from build123d import *

# Parameters (mm, degrees)
SKETCH1_R           = 1.5
SKETCH1_R_2         = 3
SKETCH1_R_3         = 12
SKETCH1_W           = 2.8
SKETCH1_H           = 30
BOSS_EXTRUDE4_DEPTH = 3


with BuildPart() as part:
    # Sketch1 → Boss-Extrude4 (new body)
    with BuildSketch(Plane(origin=(0, 0, 0), x_dir=(1, 0, 0), z_dir=(0, 1, 0))):
        with BuildLine():
            Line((-121.196449229, -126.808304592), (-11.829794241, -126.808304592))
            ThreePointArc((-11.829794241, -126.808304592), (9.383409194, -118.021508028), (18.170205759, -96.808304592))
            Line((18.170205759, -96.808304592), (18.170205759, -42.124977099))
            ThreePointArc((18.170205759, -42.124977099), (-66.513121735, 42.558350395), (-151.196449229, -42.124977099))
            Line((-151.196449229, -42.124977099), (-151.196449229, -96.808304592))
            ThreePointArc((-151.196449229, -96.808304592), (-142.409652664, -118.021508028), (-121.196449229, -126.808304592))
        make_face()
        with Locations(Location((-19.417066349, 12.133998526, 0), (0, 0, 270))):
            Circle(SKETCH1_R, mode=Mode.SUBTRACT)
        with Locations(Location((-19.417066349, -63.912266725, 0), (0, 0, 270))):
            Circle(SKETCH1_R, mode=Mode.SUBTRACT)
        with Locations(Location((-113.609177122, -63.912266725, 0), (0, 0, 270))):
            Circle(SKETCH1_R, mode=Mode.SUBTRACT)
        with Locations(Location((-113.609177122, 12.133998526, 0), (0, 0, 270))):
            Circle(SKETCH1_R, mode=Mode.SUBTRACT)
        with Locations(Location((-20.763121735, -6.941649605, 0), (0, 0, 270))):
            Circle(SKETCH1_R, mode=Mode.SUBTRACT)
        with Locations(Location((-112.263121735, -6.941649605, 0), (0, 0, 270))):
            Circle(SKETCH1_R, mode=Mode.SUBTRACT)
        with Locations(Location((-112.263121735, -51.941649605, 0), (0, 0, 270))):
            Circle(SKETCH1_R, mode=Mode.SUBTRACT)
        with Locations(Location((-66.513121735, -115.308304592, 0), (0, 0, 270))):
            Circle(SKETCH1_R_2, mode=Mode.SUBTRACT)
        with Locations(Location((8.170205759, -42.124977099, 0), (0, 0, 270))):
            Circle(SKETCH1_R, mode=Mode.SUBTRACT)
        with Locations(Location((-141.196449229, -42.124977099, 0), (0, 0, 270))):
            Circle(SKETCH1_R, mode=Mode.SUBTRACT)
        with Locations(Location((-66.513121735, 5.435278237, 0), (0, 0, 270))):
            Circle(SKETCH1_R_3, mode=Mode.SUBTRACT)
        with Locations(Location((-66.513121735, 25.558350395, 0), (0, 0, 270))):
            Circle(SKETCH1_R_2, mode=Mode.SUBTRACT)
        with Locations(Location((-66.513121735, -69.564721763, 0), (0, 0, 270))):
            Circle(SKETCH1_R_3, mode=Mode.SUBTRACT)
        with Locations(Location((-107.213121735, -116.69721419, 0), (0, 0, 270))):
            Circle(SKETCH1_R, mode=Mode.SUBTRACT)
        with Locations(Location((-25.813121735, -116.69721419, 0), (0, 0, 270))):
            Circle(SKETCH1_R, mode=Mode.SUBTRACT)
        with Locations(Location((-25.813121735, -57.29721419, 0), (0, 0, 270))):
            Circle(SKETCH1_R, mode=Mode.SUBTRACT)
        with Locations(Location((-123.013121735, -10.138406212, 0), (0, 0, 270))):
            Circle(SKETCH1_R, mode=Mode.SUBTRACT)
        with Locations(Location((-107.213121735, -57.29721419, 0), (0, 0, 270))):
            Circle(SKETCH1_R, mode=Mode.SUBTRACT)
        with Locations(Location((-114.013120412, -46.008407352, 0), (0, 0, 270))):
            Circle(SKETCH1_R, mode=Mode.SUBTRACT)
        with Locations(Location((-19.013119912, -46.008407352, 0), (0, 0, 270))):
            Circle(SKETCH1_R, mode=Mode.SUBTRACT)
        with Locations(Location((-19.013119912, -103.708406252, 0), (0, 0, 270))):
            Circle(SKETCH1_R, mode=Mode.SUBTRACT)
        with Locations(Location((-114.013120412, -103.708406252, 0), (0, 0, 270))):
            Circle(SKETCH1_R, mode=Mode.SUBTRACT)
        with Locations(Location((-10.013121735, -10.138406212, 0), (0, 0, 270))):
            Circle(SKETCH1_R, mode=Mode.SUBTRACT)
        with Locations(Location((-10.013121735, -121.478406212, 0), (0, 0, 270))):
            Circle(SKETCH1_R, mode=Mode.SUBTRACT)
        with Locations(Location((-123.013121735, -121.478406212, 0), (0, 0, 270))):
            Circle(SKETCH1_R, mode=Mode.SUBTRACT)
        with Locations(Location((-125.513121735, -116.69721419, 0), (0, 0, 270))):
            Circle(SKETCH1_R, mode=Mode.SUBTRACT)
        with Locations(Location((-125.513121735, -45.59721419, 0), (0, 0, 270))):
            Circle(SKETCH1_R, mode=Mode.SUBTRACT)
        with Locations(Location((-7.513121735, -116.69721419, 0), (0, 0, 270))):
            Circle(SKETCH1_R, mode=Mode.SUBTRACT)
        with Locations(Location((-7.513121735, -45.59721419, 0), (0, 0, 270))):
            Circle(SKETCH1_R, mode=Mode.SUBTRACT)
        with Locations(Location((-80.013121735, 38.378834062, 0), (0, 0, 270))):
            Circle(SKETCH1_R, mode=Mode.SUBTRACT)
        with Locations(Location((-80.013121735, -19.621165938, 0), (0, 0, 270))):
            Circle(SKETCH1_R, mode=Mode.SUBTRACT)
        with Locations(Location((-31.013121735, -19.621165938, 0), (0, 0, 270))):
            Circle(SKETCH1_R, mode=Mode.SUBTRACT)
        with Locations(Location((-27.513121735, -72.508406212, 0), (0, 0, 270))):
            Circle(SKETCH1_R, mode=Mode.SUBTRACT)
        with Locations(Location((-27.513121735, -121.508406212, 0), (0, 0, 270))):
            Circle(SKETCH1_R, mode=Mode.SUBTRACT)
        with Locations(Location((-85.513121735, -72.508406212, 0), (0, 0, 270))):
            Circle(SKETCH1_R, mode=Mode.SUBTRACT)
        with Locations(Location((-85.513121735, -121.508406212, 0), (0, 0, 270))):
            Circle(SKETCH1_R, mode=Mode.SUBTRACT)
        with Locations(Location((-42.013121735, -100.008406212, 0), (0, 0, 270))):
            Circle(SKETCH1_R, mode=Mode.SUBTRACT)
        with Locations(Location((-91.013121735, -100.008406212, 0), (0, 0, 270))):
            Circle(SKETCH1_R, mode=Mode.SUBTRACT)
        with Locations(Location((-42.013121735, -42.008406212, 0), (0, 0, 270))):
            Circle(SKETCH1_R, mode=Mode.SUBTRACT)
        with Locations(Location((-91.013121735, -42.008406212, 0), (0, 0, 270))):
            Circle(SKETCH1_R, mode=Mode.SUBTRACT)
        with Locations(Location((-66.513121735, -109.124977099, 0), (0, 0, 270))):
            Circle(SKETCH1_R, mode=Mode.SUBTRACT)
        with Locations(Location((-66.513121735, -24.124977099, 0), (0, 0, 270))):
            Circle(SKETCH1_R, mode=Mode.SUBTRACT)
        with Locations(Location((-24.013121735, -66.624977099, 0), (0, 0, 270))):
            Circle(SKETCH1_R, mode=Mode.SUBTRACT)
        with Locations(Location((-109.013121735, -66.624977099, 0), (0, 0, 270))):
            Circle(SKETCH1_R, mode=Mode.SUBTRACT)
        with Locations(Location((-141.196449229, -109.124977099, 0), (0, 0, 270))):
            Circle(SKETCH1_R, mode=Mode.SUBTRACT)
        with Locations(Location((8.170205759, -109.124977099, 0), (0, 0, 270))):
            Circle(SKETCH1_R, mode=Mode.SUBTRACT)
        with Locations(Location((-20.763121735, -51.941649605, 0), (0, 0, 270))):
            Circle(SKETCH1_R, mode=Mode.SUBTRACT)
        with BuildLine():
            Line((-139.496449229, -88.862296701), (-139.496449229, -62.387657497))
            ThreePointArc((-139.496449229, -62.387657497), (-141.196449229, -60.687657497), (-142.896449229, -62.387657497))
            Line((-142.896449229, -62.387657497), (-142.896449229, -88.862296701))
            ThreePointArc((-142.896449229, -88.862296701), (-141.196449229, -90.562296701), (-139.496449229, -88.862296701))
        make_face(mode=Mode.SUBTRACT)
        with BuildLine():
            Line((-78.513121735, -120.108304592), (-54.513121735, -120.108304592))
            ThreePointArc((-54.513121735, -120.108304592), (-52.813121735, -121.808304592), (-54.513121735, -123.508304592))
            Line((-54.513121735, -123.508304592), (-78.513121735, -123.508304592))
            ThreePointArc((-78.513121735, -123.508304592), (-80.213121735, -121.808304592), (-78.513121735, -120.108304592))
        make_face(mode=Mode.SUBTRACT)
        with Locations((-14.413121735, -25.911649605)):
            Rectangle(SKETCH1_W, SKETCH1_H, mode=Mode.SUBTRACT)
        with Locations((-118.613121735, -25.911649605)):
            Rectangle(SKETCH1_W, SKETCH1_H, mode=Mode.SUBTRACT)
        with BuildLine():
            Line((9.870205759, -88.862296701), (9.870205759, -62.387657497))
            ThreePointArc((9.870205759, -62.387657497), (8.170205759, -60.687657497), (6.470205759, -62.387657497))
            Line((6.470205759, -62.387657497), (6.470205759, -88.862296701))
            ThreePointArc((6.470205759, -88.862296701), (8.170205759, -90.562296701), (9.870205759, -88.862296701))
        make_face(mode=Mode.SUBTRACT)
    extrude(amount=BOSS_EXTRUDE4_DEPTH)


solid = part.part
Can you work these out from the model? Positions are in its coordinate system, mm. Round coordinates to 2 decimals unless told otherwise and drop trailing zeros. Order: outer loops, then holes, each group sorted by start corner. A loop starts at its lowest first (then second) coordinate and runs counter-clockwise, first axis right, second up. Notation, with made-up numbers: M 73.25,83 L 98.25,83 A16 ccw 98.25,108 Z; hole C 29,-4 d2. An arc over 180 degrees is marked long. Use a Markdown table: item, result.
1) If we mould it in two halves opening along Z, with no side actions, what happens to faces 1 (the face through (9.1, 1.5, 118.3)), 2 (the face through (-78.228, 1.479, -8.037)), 3 (the face through (-68, 3, 41)), 4 (the face through (-71.11, 1.48, 80.65))? For each: +Z half, -Z half, draft (parallel to the pull), parting line (faces both ways), or undercut.
Geometry says:
| item | result |
|---|---|
| face 1 | +Z half |
| face 2 | undercut |
| face 3 | draft |
| face 4 | undercut |
2) Imagine slicing it at C-C (x = -37). List the corners of the cut face in (y, z) for me.
Geometry says:
| item | result |
|---|---|
| outline | M 0,-37.25 L 3,-37.25 L 3,126.81 L 0,126.81 Z |
3) I'm going to push flat-ended pins straight in: P1, Ø0.9, axis at y = 1, z = 21, coming from the -X side; P2, Ø2.5, axis at x = -141.2, z = 42.12, coming from the -Y side; P3, Ø0.9, axis at y = 1.5, z = 28.5, coming from the +X side; P4, Ø1.5, axis at x = -34, y = 2, coming from the -Z side. Where does each tip first touch, or does it pass through?
Geometry says:
| item | result |
|---|---|
| P1 | stops at x = -148.63 |
| P2 | passes through |
| P3 | stops at x = 17.14 |
| P4 | stops at z = -36.38 |
4) Imagine slicing it at D-D (x = 3.5). List the corners of the cut face in (y, z) for me.
Geometry says:
| item | result |
|---|---|
| outline | M 0,-5.51 L 3,-5.51 L 3,122.6 L 0,122.6 Z |
5) Imagine slicing it at B-B (y = 1.2). Give the number of separate pieces and of enclosed holes in the cut face, then the cut area to 3 significant figures.
Geometry says:
| item | result |
|---|---|
| separate pieces | 1 |
| enclosed holes | 52 |
| area | 23,500 mm² |
6) If I drill on line 1 along X through (y, z) = (2.8, 87.5); line 2 along Z through (x, y) = (-58, 2.1); line 3 along X through (y, z) = (1.5, 66), over which ranges is the centre line in solid material (lowest first)?
Geometry says:
| item | result |
|---|---|
| line 1 | x = -151.2 to -142.9, -139.5 to 6.47, 9.87 to 18.17 |
| line 2 | z = -42.13 to -13.89, 3.02 to 61.11, 78.02 to 120.11, 123.51 to 126.81 |
| line 3 | x = -151.2 to -142.9, -139.5 to -110.38, -107.65 to -77.97, -55.05 to -25.38, -22.65 to 6.47, 9.87 to 18.17 |
7) Imagine slicing it at A-A (x = -59). List the corners of the cut face in (y, z) for me, then the cut area to 3 significant figures.
Geometry says:
| item | result |
|---|---|
| outline | M 0,-42.22 L 3,-42.22 L 3,-14.79 L 0,-14.79 Z; M 0,3.92 L 3,3.92 L 3,60.21 L 0,60.21 Z; M 0,78.92 L 3,78.92 L 3,120.11 L 0,120.11 Z; M 0,123.51 L 3,123.51 L 3,126.81 L 0,126.81 Z |
| area | 385 mm² |
